```python
from build123d import *

# Parameters (mm, degrees)
F0_W     = 406.4
F0_H     = 609.6
F1_DEPTH = 203.2
F2_W     = 246.5967833996
F2_H     = 524.6225595474
F3_DEPTH = 196.85
F4_W     = 524.6225595474
F4_H     = 175.7622616529
F5_DEPTH = 107.4888
F6_W     = 406.4
F6_H     = 609.6
F6_W_2   = 246.5967833996
F6_H_2   = 524.6225595474
F7_DEPTH = 25.4


with BuildPart() as f1:
    # F0 (on Top) → F1 (new body)
    with BuildSketch(Plane.XY):
        Rectangle(F0_W, F0_H)
    extrude(amount=F1_DEPTH)

    # F2 (on face) → F3 (cut)
    with BuildSketch(Plane.XY.offset(203.2)):
        with Locations((-51.9739538431, 8.2974731922)):
            Rectangle(F2_W, F2_H)
    extrude(amount=-F3_DEPTH, mode=Mode.SUBTRACT)

    # F4 (on face) → F5 (cut)
    with BuildSketch(Plane(origin=(71.3244378567, 0, 0), x_dir=(0, -1, 0), z_dir=(-1, 0, 0))):
        with Locations((-8.2974731922, 94.2311308265)):
            Rectangle(F4_W, F4_H)
    extrude(amount=-F5_DEPTH, mode=Mode.SUBTRACT)

    # F6 (on face) → F7 (join)
    with BuildSketch(Plane.XY.offset(203.2)):
        Rectangle(F6_W, F6_H)
        with Locations((-51.9739538431, 8.2974731922)):
            Rectangle(F6_W_2, F6_H_2, mode=Mode.SUBTRACT)
        with BuildLine():
            ThreePointArc((132.4002933692, 174.6901672035), (132.4002933677, 174.6900416756), (132.4002933629, 174.6899161476))
            Line((132.4002933629, 174.6899161476), (132.3993421334, 136.9216628493))
            ThreePointArc((132.3993421334, 136.9216628493), (127.4147392292, 131.9386900836), (122.4331459754, 136.924671667))
            Line((122.4331459754, 136.924671667), (122.4547239005, 174.2168030567))
            ThreePointArc((122.4547239005, 174.2168030567), (127.1792936349, 179.66858125), (132.4002933692, 174.6901672035))
        make_face(mode=Mode.SUBTRACT)
        with BuildLine():
            ThreePointArc((132.8256002304, 232.8666895628), (132.8256002288, 232.8665640349), (132.8256002241, 232.866438507))
            Line((132.8256002241, 232.866438507), (132.8246489946, 195.0981852086))
            ThreePointArc((132.8246489946, 195.0981852086), (127.8400460904, 190.115212443), (122.8584528366, 195.1011940263))
            Line((122.8584528366, 195.1011940263), (122.8800307617, 232.393325416))
            ThreePointArc((122.8800307617, 232.393325416), (127.6046004961, 237.8451036093), (132.8256002304, 232.8666895628))
        make_face(mode=Mode.SUBTRACT)
    extrude(amount=F7_DEPTH)


solid = f1.part
```
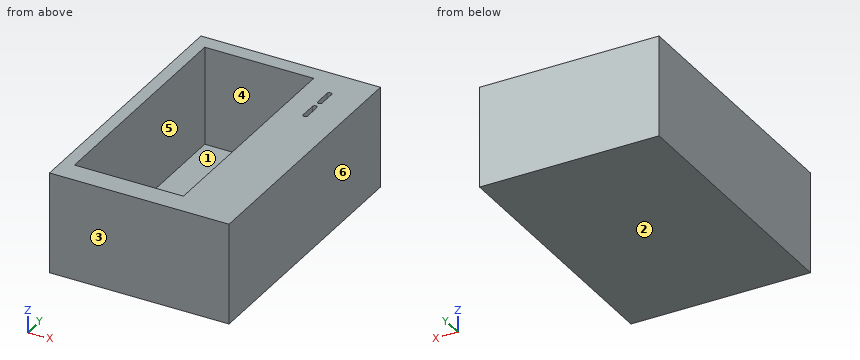
Geometry: final body of the model. Coordinates: model frame, mm. Face numbers are marked on the shaded views. A direction names the side the tool comes from. Give positions to 0.01 mm unless a question says otherwise; leave off trailing zeros. Loops run counter-clockwise (first coordinate to the right, second up) from the corner with the lowest first, then second, coordinate; pieces in that order, holes last. Notation, with made-up numbers: (68.25, 80) - (113.25, 80) arc R11 ccw to (113.25, 86) - close; hole circle Ø8 at (82.5, 78.5). An arc over 180 degrees is marked (long way). Answer as CSV lines item,"result". Start each with the question number.
(1) Reachability of the marked faces 1 and 2 from +Z, -Z, +X, -X, +Y, -Y: full face, straight path, thin tool, end or side. Return the list, or none.
(2) Section query A-A (z = 90). Output: boundary loops of the cut face in (x, y).
(3) Mould query, pull axis Y, two halves, no side actions, for the marked faces 3, 4, 5 and 6. Classes: +Y half, -Y half, draft (parallel to the pull), parting line (faces both ways), or undercut.
(4) Section query C-C (y = 249). Output: boundary loops of the cut face in (x, z), and give its area (3 significant figures).
(5) Pin query (flat end, axial travel): P1, Ø5, axis at x = 127, y = 157, coming from the +Z side; P2, Ø4, axis at x = 54.5, y = 21, coming from the +Z side. Return the tip coordinate at first contact, or that it passes through.
(6) Ray query, line 1 along Y through (x, z) = (-134, 109); line 2 along X through (y, z) = (-153.5, 37); line 3 along Z through (x, y) = (130.5, 23.5). Return the intervals inside material, ascending. Write a range as [from, to].
(7) Section query B-B (x = 104). Output: boundary loops of the cut face in (y, z), and give its area (3 significant figures).
(8) Section query D-D (x = -3). Output: boundary loops of the cut face in (y, z).
Worked answers:
1,face 1,"none"
1,face 2,"-Z, +X, -X, +Y, -Y"
2,outline,"(-203.2, -304.8) - (203.2, -304.8) - (203.2, 304.8) - (-203.2, 304.8) - close; hole (-175.27, -254.01) - (178.81, -254.01) - (178.81, 270.61) - (-175.27, 270.61) - close"
3,face 3,"-Y half"
3,face 4,"undercut"
3,face 5,"undercut"
3,face 6,"draft"
4,outline,"(-203.2, 0) - (203.2, 0) - (203.2, 228.6) - (71.32, 228.6) - (71.32, 182.11) - (178.81, 182.11) - (178.81, 6.35) - (-175.27, 6.35) - (-175.27, 228.6) - (-203.2, 228.6) - close"
4,area,"19,200 mm^2"
5,P1,"stops at z = 203.2"
5,P2,"stops at z = 6.35"
6,line 1,"y = [-304.8, -254.01], [270.61, 304.8]"
6,line 2,"x = [-203.2, -175.27], [178.81, 203.2]"
6,line 3,"z = [0, 6.35], [182.11, 228.6]"
7,outline,"(-304.8, 0) - (304.8, 0) - (304.8, 228.6) - (-304.8, 228.6) - close; hole (-254.01, 6.35) - (270.61, 6.35) - (270.61, 182.11) - (-254.01, 182.11) - close"
7,area,"47,100 mm^2"
8,outline,"(-304.8, 0) - (304.8, 0) - (304.8, 228.6) - (270.61, 228.6) - (270.61, 6.35) - (-254.01, 6.35) - (-254.01, 228.6) - (-304.8, 228.6) - close"
